```python
from build123d import *

# Parameters (mm, degrees)
F0_W        = 195
F0_H        = 195
F1_DEPTH    = 4.0000047
F2_T1_DEPTH = 247.2565983155
F3_T1_DEPTH = 247.2565983155
F4_T1_DEPTH = 226.9365983155


# Not quite as in the source:
# - a fillet or chamfer that OpenCascade refuses, or shapes differently, is made with other operations: its cross-section is extruded or revolved along the edge and cut away or added


with BuildPart() as f1:
    # F0 (on Front) → F1 (new body, symmetric)
    with BuildSketch(Plane.XZ):
        Rectangle(F0_W, F0_H)
    extrude(amount=F1_DEPTH, both=True)

    # F2: chamfer of 10.16 on 1 edges, made by hand

    # F2_s2 → F2_t1 (cut)
    with BuildSketch(Plane.XY.offset(-123.6282991577)):
        Polygon((97.5, 6.1599953), (87.34, -4.0000047), (97.5, -4.0000047), align=None)
    extrude(amount=F2_T1_DEPTH, mode=Mode.SUBTRACT)

    # F3: chamfer of 10.16 on 1 edges, made by hand

    # F3_s2 → F3_t1 (cut)
    with BuildSketch(Plane.XY.offset(-123.6282991577)):
        Polygon((-97.5, 6.1599953), (-87.34, -4.0000047), (-97.5, -4.0000047), align=None)
    extrude(amount=F3_T1_DEPTH, mode=Mode.SUBTRACT)

    # F4: chamfer of 10.16 on 1 edges, made by hand

    # F4_s2 → F4_t1 (cut)
    with BuildSketch(Plane.YZ.offset(-113.4682991577)):
        Polygon((6.1599953, 97.5), (-4.0000047, 87.34), (-4.0000047, 97.5), align=None)
    extrude(amount=F4_T1_DEPTH, mode=Mode.SUBTRACT)


solid = f1.part
```
Verification items for the finished model (mm, model axes). Give positions to 0.01 mm unless a question says otherwise; leave off trailing zeros. Write each loop counter-clockwise with the first axis right and the second up, starting at its lowest first coordinate (ties: lowest second). Pieces come first, ordered by that corner, then holes. Notation, with made-up numbers: (70.25, 6) - (86.25, 6) arc R11 cw to (86.25, 24) - close; hole circle Ø7 at (-38.5, -0.5). An arc over 180 degrees is marked (long way). Put each result on its own line as item: value.
Q1. Scan lines: probe 1 along Z at (x, y) = (79, -3.5); probe 2 along X at (y, z) = (-2, -13.5); probe 3 along X at (y, z) = (-0.25, 13.5). Record each from-to range of solid material in increasing order. Write a range as from..to.
Result:
probe 1: -97.5..87.84
probe 2: -89.34..89.34
probe 3: -91.09..91.09
Q2. Depth check by flat-ended pin: P1, Ø1, axis at x = -33, y = 0.5, coming from the +Z side; P2, Ø4, axis at y = -3, z = 35, coming from the +X side. Enter the tip coordinate at first touch or a pass-through.
Result:
P1: z = 92.34
P2: x = 90.34
Q3. Section check A-A on y = 0. Record the cut outline in (x, z).
Result:
outline: (-91.34, -97.5) - (91.34, -97.5) - (91.34, 91.34) - (-91.34, 91.34) - close
Q4. Section check B-B on x = 34.5. Record the cut outline in (y, z).
Result:
outline: (-4, -97.5) - (4, -97.5) - (4, 95.34) - (-4, 87.34) - close
